Read the model definition and answer for the solid it produces. Units are mm, in the model's axes. A direction names the side the tool comes from. Give positions to 0.01 mm unless a question says otherwise; leave off trailing zeros. Loops run counter-clockwise (first coordinate to the right, second up) from the corner with the lowest first, then second, coordinate; pieces in that order, holes last. Notation, with made-up numbers: (6, 56) - (26, 56) arc R16 cw to (26, 70) - close; hole circle Ø6 at (44, 60). An arc over 180 degrees is marked (long way). Use a Markdown table: item, result. Add a question column.
Item 1: A cutting plane is placed at D-D (x = 25). Determine the outline of the cut face in (y, z) (3 decimals).
Item 2: Each of these flat-tipped pins is pushed along its axis until it touches: P1, Ø7, axis at x = -25, z = -2.5, coming from the +Y side; P2, Ø8, axis at x = 17.78, z = -30.8, coming from the -Y side; P3, Ø4, axis at y = 3, z = -7, coming from the +X side. Where does it stop, or does it pass through?
Item 3: A cutting plane is placed at C-C (z = 0). Give the number of separate pieces and of enclosed holes in the cut face, plus the area to 3 significant figures.
Item 4: A cutting plane is placed at A-A (x = 0). Determine the outline of the cut face in (y, z) (3 decimals), plus the area to 3 significant figures.
Item 5: A cutting plane is placed at B-B (y = -2.5). Determine the outline of the cut face in (x, z).
Item 6: Consider probe 1 along X at (y, z) = (1.2, 0); probe 2 along Z at (x, y) = (-2.5, 6.25); probe 3 along Z at (x, y) = (-25, 0.7). Determine where each line is inside the solid, lowest interval first. Write a range as [from, to].
Item 7: For a pull along Z with two mould halves and no side action, classify faces 1 (the face through (28, 0, 12)), 2 (the face through (-40, 3, -9)), 3 (the face through (-17.6, 2.7, -26.3)) as +Z half, -Z half, draft (parallel to the pull), parting line (faces both ways), or undercut.
Item 8: Which of the six approach directions +Z, -Z, +X, -X, +Y, -Y give full straight-line access (tool end or side, diameter ignored) to faces 4 (the face through (-2.82, -2.26, -23.49)), 5 (the face through (-39.95, 2.71, 0.98)), 6 (the face through (-18.546, 4.841, -3.357))?
from build123d import *

# Parameters (mm, degrees)
SKETCH1_R                               = 41
BOSS_EXTRUDE1_DEPTH                     = 7
CBORE_FOR_M6_HEX_HEAD_BOLT1_D           = 6.4
CBORE_FOR_M6_HEX_HEAD_BOLT1_CBORE_D     = 14.55
CBORE_FOR_M6_HEX_HEAD_BOLT1_CBORE_DEPTH = 4.38
CIRPATTERN2_COUNT                       = 4
CUT_EXTRUDE4_START                      = -7
SKETCH15_R                              = 2.5
CUT_EXTRUDE4_DEPTH                      = 66.403767002
SKETCH16_R                              = 4.5
CUT_EXTRUDE5_DEPTH                      = 5.5
BOSS_EXTRUDE2_START                     = 7
SKETCH17_R                              = 30
SKETCH17_R_2                            = 3.2
BOSS_EXTRUDE2_DEPTH                     = 7


with BuildPart() as part:
    # Sketch1 → Boss-Extrude1 (new body)
    with BuildSketch(Plane(origin=(0, 0, 0), x_dir=(1, 0, 0), z_dir=(0, 1, 0))):
        with Locations(Location((0, 0, 0), (0, 0, 270))):
            Circle(SKETCH1_R)
    extrude(amount=BOSS_EXTRUDE1_DEPTH)

    # CBORE for M6 Hex Head Bolt1 (through all)
    with Locations(Plane(origin=(0, 7, 0), x_dir=(1, 0, 0), z_dir=(0, 1, 0))):
        with Locations((0, 25)):
            cbore_for_m6_hex_head_bolt1 = CounterBoreHole(CBORE_FOR_M6_HEX_HEAD_BOLT1_D / 2, CBORE_FOR_M6_HEX_HEAD_BOLT1_CBORE_D / 2, CBORE_FOR_M6_HEX_HEAD_BOLT1_CBORE_DEPTH)

    # CirPattern2: CBORE for M6 Hex Head Bolt1 ×4 about axis
    cirpattern2_axis = Axis((0, 0, 0), (0, 1, 0))
    for i in range(1, CIRPATTERN2_COUNT):
        add(cbore_for_m6_hex_head_bolt1.rotate(cirpattern2_axis, i * 360 / CIRPATTERN2_COUNT), mode=Mode.SUBTRACT)

    # Sketch15 → Cut-Extrude4 (cut, through all)
    with BuildSketch(Plane.XZ.offset(CUT_EXTRUDE4_START)):
        with Locations(Location((35.56, 0, 0), (0, 0, 90))):
            Circle(SKETCH15_R)
        with Locations(Location((17.78, -30.795863359, 0), (0, 0, 90))):
            Circle(SKETCH15_R)
        with Locations(Location((-17.78, -30.795863359, 0), (0, 0, 90))):
            Circle(SKETCH15_R)
        with Locations(Location((-35.56, 0, 0), (0, 0, 90))):
            Circle(SKETCH15_R)
        with Locations(Location((-17.78, 30.795863359, 0), (0, 0, 90))):
            Circle(SKETCH15_R)
    extrude(amount=CUT_EXTRUDE4_DEPTH, mode=Mode.SUBTRACT)

    # Sketch16 → Cut-Extrude5 (cut)
    with BuildSketch(Plane.XZ):
        with Locations(Location((-17.78, 30.795863359, 0), (0, 0, 270))):
            Circle(SKETCH16_R)
        with Locations(Location((-35.56, 0, 0), (0, 0, 270))):
            Circle(SKETCH16_R)
        with Locations(Location((35.56, 0, 0), (0, 0, 270))):
            Circle(SKETCH16_R)
        with Locations(Location((-17.78, -30.795863359, 0), (0, 0, 270))):
            Circle(SKETCH16_R)
        with Locations(Location((17.78, -30.795863359, 0), (0, 0, 270))):
            Circle(SKETCH16_R)
    extrude(amount=-CUT_EXTRUDE5_DEPTH, mode=Mode.SUBTRACT)

    # Sketch17 → Boss-Extrude2 (add)
    with BuildSketch(Plane.XZ.offset(BOSS_EXTRUDE2_START)):
        with Locations(Location((0, 0, 0), (0, 0, 90))):
            Circle(SKETCH17_R)
        with Locations(Location((25, 0, 0), (0, 0, 90))):
            Circle(SKETCH17_R_2, mode=Mode.SUBTRACT)
        with Locations(Location((0, -25, 0), (0, 0, 90))):
            Circle(SKETCH17_R_2, mode=Mode.SUBTRACT)
        with Locations(Location((-25, 0, 0), (0, 0, 90))):
            Circle(SKETCH17_R_2, mode=Mode.SUBTRACT)
        with Locations(Location((0, 25, 0), (0, 0, 90))):
            Circle(SKETCH17_R_2, mode=Mode.SUBTRACT)
    extrude(amount=-BOSS_EXTRUDE2_DEPTH)


solid = part.part
Geometry says:
| question | item | result |
|---|---|---|
| 1 | outline | (-7, -16.583) - (0, -16.583) - (0, -32.496) - (7, -32.496) - (7, -7.275) - (2.62, -7.275) - (2.62, -3.2) - (-7, -3.2) - close; (-7, 3.2) - (2.62, 3.2) - (2.62, 7.275) - (7, 7.275) - (7, 32.496) - (0, 32.496) - (0, 16.583) - (-7, 16.583) - close |
| 2 | P1 | y = 2.62 |
| 2 | P2 | y = 5.5 |
| 2 | P3 | x = 40.69 |
| 3 | separate pieces | 7 |
| 3 | enclosed holes | 0 |
| 3 | area | 636 mm² |
| 4 | outline | (-7, -30) - (0, -30) - (0, -41) - (7, -41) - (7, -32.275) - (2.62, -32.275) - (2.62, -28.2) - (-7, -28.2) - close; (-7, -21.8) - (2.62, -21.8) - (2.62, -17.725) - (7, -17.725) - (7, 17.725) - (2.62, 17.725) - (2.62, 21.8) - (-7, 21.8) - close; (-7, 28.2) - (2.62, 28.2) - (2.62, 32.275) - (7, 32.275) - (7, 41) - (0, 41) - (0, 30) - (-7, 30) - close |
| 4 | area | 743 mm² |
| 5 | outline | circle Ø60 at (0, 0); hole circle Ø6.4 at (-25, 0); hole circle Ø6.4 at (0, -25); hole circle Ø6.4 at (0, 25); hole circle Ø6.4 at (25, 0) |
| 6 | probe 1 | [-41, -40.06], [-31.06, -28.2], [-21.8, 21.8], [28.2, 31.06], [40.06, 41] |
| 6 | probe 2 | [-40.92, -31.83], [-18.17, 18.17], [31.83, 40.92] |
| 6 | probe 3 | [-32.5, -3.2], [3.2, 32.5] |
| 7 | face 1 | draft |
| 7 | face 2 | parting line |
| 7 | face 3 | undercut |
| 8 | face 4 | +Y, -Y |
| 8 | face 5 | -Y |
| 8 | face 6 | +Y |
